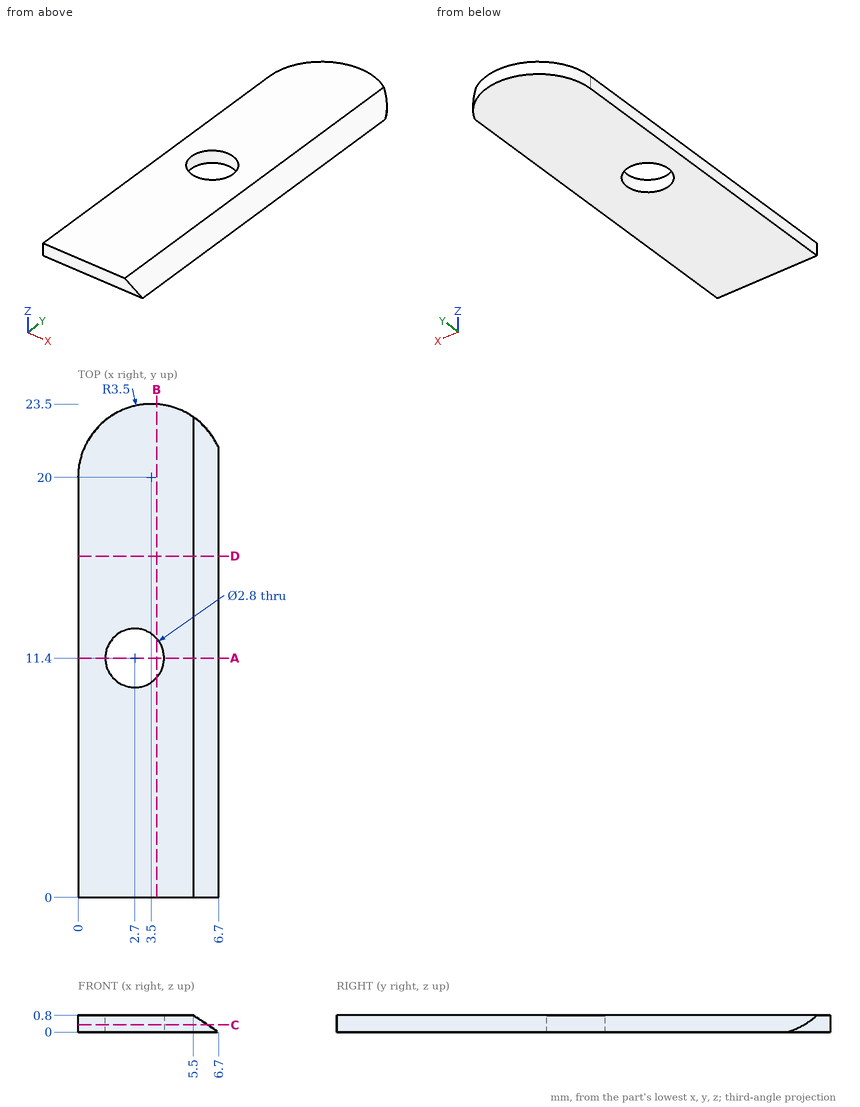
Design review of the part shown in the three views and the two pictorial views. Dimensions are in mm from the part's minimum x, y and z. Give positions to 0.01 mm unless a question says otherwise; leave off trailing zeros. Loops run counter-clockwise (first coordinate to the right, second up) from the corner with the lowest first, then second, coordinate; pieces in that order, holes last. Notation, with made-up numbers: M 65.25,-13.5 L 112.25,-13.5 A20 cw 112.25,-8.5 Z; hole C 70,51.5 d3. An arc over 180 degrees is marked long. Answer as a JSON object with one key per item and string values. Group by question number.
Q1. For probe 1 along Y at (x, z) = (2.5, 0.3); probe 2 along Y at (x, z) = (3, 0.2); probe 3 along Z at (x, y) = (6.25, 22), list the stretches that pass through material, from the lowest coordinate up. Write a range as [from, to].
Q2. Add section B-B on x = 3.75. Give the boundary of the cut face in (y, z).
Q3. Add section A-A on y = 11.4. Give the boundary of the cut face in (x, z).
Q4. Add section C-C on z = 0.35. Give the boundary of the cut face in (x, y) (3 decimals), and give its area (3 significant figures).
Q5. Add section D-D on y = 16.25. Give the boundary of the cut face in (x, z), and give its area (3 significant figures).
Q6. Insertion check: P1, Ø2, axis at x = 2.7, y = 11.4, coming from the -Z side. The pin has a flat end and moves straight along its axis. Give the tip position at first contact, or say it passes through.
Checked values:
{
 "1": {"probe 1": "[0, 10.01], [12.79, 23.35]", "probe 2": "[0, 10.03], [12.77, 23.46]", "probe 3": "[0, 0.3]"},
 "2": {"outline": "M 0,0 L 10.47,0 L 10.47,0.8 L 0,0.8 Z; M 12.33,0 L 23.49,0 L 23.49,0.8 L 12.33,0.8 Z"},
 "3": {"outline": "M 0,0 L 1.3,0 L 1.3,0.8 L 0,0.8 Z; M 4.1,0 L 6.7,0 L 5.5,0.8 L 4.1,0.8 Z"},
 "4": {"outline": "M 0,0 L 6.175,0 L 6.175,22.257 A3.5 ccw 0,20 Z; hole C 2.7,11.4 d2.8", "area": "135 mm²"},
 "5": {"outline": "M 0,0 L 6.7,0 L 5.5,0.8 L 0,0.8 Z", "area": "4.88 mm²"},
 "6": {"P1": "through"}
}
